```python
from build123d import *

# Parameters (mm, degrees)
F1_DEPTH  = 72
F2_W      = 201
F2_H      = 39
F3_DEPTH  = 4
F5_DEPTH  = 4
F6_R      = 2
F7_W      = 7
F7_H      = 7
F8_DEPTH  = 22
F9_W      = 7
F9_H      = 7
F10_DEPTH = 80
F11_R     = 2


with BuildPart() as f1:
    # F0 (on Front) → F1 (new body)
    with BuildSketch(Plane.XZ):
        Polygon((-92.8763775631, 18.0203217369), (-94.8763775631, 18.0203217369), (-94.8763775631, -16.9746782631), (-90.8713775631, -20.9796782631), (102.1186224369, -20.9796782631), (106.1236224369, -16.9746782631), (106.1236224369, 18.0203217369), (104.1236224369, 18.0203217369), (104.1236224369, -16.1462511383), (101.2901953121, -18.9796782631), (-90.0429504384, -18.9796782631), (-92.8763775631, -16.1462511383), align=None)
    extrude(amount=F1_DEPTH)

    # F2 (on face) → F3 (join)
    with BuildSketch(Plane(origin=(0, 0, 0), x_dir=(-1, 0, 0), z_dir=(0, 1, 0))):
        with Locations((-5.6236224369, -1.4796782631)):
            Rectangle(F2_W, F2_H)
    extrude(amount=F3_DEPTH)

    # F4 (on face) → F5 (join)
    with BuildSketch(Plane.XZ.offset(72)):
        Polygon((106.1236224369, 18.0203217369), (-94.8763775631, 18.0203217369), (-94.8763775631, -16.9746782631), (-90.8713775631, -20.9796782631), (102.1186224369, -20.9796782631), (106.1236224369, -16.9746782631), align=None)
    extrude(amount=F5_DEPTH)

    # F6
    f6_edges = [f1.edges().sort_by_distance(p)[0] for p in [
        (-94.876378, -76, 0.522822),
        (106.123622, -76, 0.522822),
    ]]
    fillet(f6_edges, radius=F6_R)

    # F7 (on face) → F8 (join)
    with BuildSketch(Plane.XZ.offset(76)):
        with Locations((49.1236224369, -1.4796782631)):
            Rectangle(F7_W, F7_H)
        with Locations((-37.8763775631, -1.4796782631)):
            Rectangle(F7_W, F7_H)
    extrude(amount=F8_DEPTH)

    # F9 (on face) → F10 (join)
    with BuildSketch(Plane.YZ.offset(-34.3763775631)):
        with Locations((-94.5, -1.4796782631)):
            Rectangle(F9_W, F9_H)
    extrude(amount=F10_DEPTH)

    # F11
    f11_edges = [f1.edges().sort_by_distance(p)[0] for p in [
        (5.623622, -98, 2.020322),
        (5.623622, -98, -4.979678),
        (5.623622, -91, 2.020322),
        (5.623622, -91, -4.979678),
    ]]
    fillet(f11_edges, radius=F11_R)


solid = f1.part
```
Design review of the part built by this model. Coordinates are the model's own, in mm. A direction names the side the tool comes from. Give positions to 0.01 mm unless a question says otherwise; leave off trailing zeros. Order: outer loops, then holes, each group sorted by start corner. A loop starts at its lowest first (then second) coordinate and runs counter-clockwise, first axis right, second up. Notation, with made-up numbers: (-32, 27) - (25, 27) arc R21 cw to (25, 54) - close; hole circle Ø2 at (42.5, -6.75). An arc over 180 degrees is marked (long way). Use a Markdown table: item, result. Add a question column.
(1) Add section C-C on z = 15. Give the boundary of the cut face in (x, y), then the cut area to 3 significant figures.
(2) Add section B-B on y = -79. Give the boundary of the cut face in (x, z), then the cut area to 3 significant figures.
(3) Add section D-D on y = -51.5. Give the boundary of the cut face in (x, z), then the cut area to 3 significant figures.
(4) Mouldability with a two-part tool opening along Y and no side actions: class faces 1 (the face through (7, -35, -18.98)), 2 (the face through (-92.9, -37.47, -18.95)), 3 (the face through (-94, 0, -20)) as +Y half, -Y half, draft (parallel to the pull), parting line (faces both ways), or undercut.
(5) Add section A-A on x = 18. Give the boundary of the cut face in (y, z).
(6) Clearance check with flat-ended pins moving along their axes: P1, Ø16, axis at x = -8, y = -88, coming from the -Z side; P2, Ø5, axis at x = 83, z = 11.5, coming from the -Y side; P3, Ø5.5, axis at y = -86.5, z = -0.5, coming from the +X side. State where each tip first meets the part, or that it passes through.
(7) Wall thickness on probe 1 along Y at (x, z) = (-21.5, -11); probe 2 along X at (y, z) = (-50, -7.5); probe 3 along Z at (x, y) = (67.5, -42): over which ranges is each line inside the solid? List them lowest first. Write a range as [from, to].
(8) Machinability: for faces 4 (the face through (-92.876, -35, 1)), 5 (the face through (52.624, -87, -2)), 6 (the face through (-41.376, -87, -2)), which of the approach directions +Z, -Z, +X, -X, +Y, -Y give a long, thin tool a straight path to every point of the face, cutting with its end or side? Answer none if there is none.
Report:
| question | item | result |
|---|---|---|
| 1 | outline | (-94.88, -74) arc R2 ccw to (-92.88, -76) - (104.12, -76) arc R2 ccw to (106.12, -74) - (106.12, 4) - (-94.88, 4) - close; hole (-92.88, -72) - (104.12, -72) - (104.12, 0) - (-92.88, 0) - close |
| 1 | area | 1,890 mm² |
| 2 | outline | (-41.38, -4.98) - (-34.38, -4.98) - (-34.38, 2.02) - (-41.38, 2.02) - close; (45.62, -4.98) - (52.62, -4.98) - (52.62, 2.02) - (45.62, 2.02) - close |
| 2 | area | 98.0 mm² |
| 3 | outline | (-94.88, -16.97) - (-90.87, -20.98) - (102.12, -20.98) - (106.12, -16.97) - (106.12, 18.02) - (104.12, 18.02) - (104.12, -16.15) - (101.29, -18.98) - (-90.04, -18.98) - (-92.88, -16.15) - (-92.88, 18.02) - (-94.88, 18.02) - close |
| 3 | area | 542 mm² |
| 4 | face 1 | undercut |
| 4 | face 2 | draft |
| 4 | face 3 | -Y half |
| 5 | outline | (-98, -2.98) arc R2 ccw to (-96, -4.98) - (-93, -4.98) arc R2 ccw to (-91, -2.98) - (-91, 0.02) arc R2 ccw to (-93, 2.02) - (-96, 2.02) arc R2 ccw to (-98, 0.02) - close; (-76, -20.98) - (4, -20.98) - (4, 18.02) - (0, 18.02) - (0, -18.98) - (-72, -18.98) - (-72, 18.02) - (-76, 18.02) - close |
| 6 | P1 | stops at z = -4.98 |
| 6 | P2 | stops at y = -76 |
| 6 | P3 | stops at x = 52.62 |
| 7 | probe 1 | y = [-76, -72], [0, 4] |
| 7 | probe 2 | x = [-94.88, -92.88], [104.12, 106.12] |
| 7 | probe 3 | z = [-20.98, -18.98] |
| 8 | face 4 | +Z |
| 8 | face 5 | +Z, -Z, +X, -Y |
| 8 | face 6 | +Z, -Z, -X, -Y |
